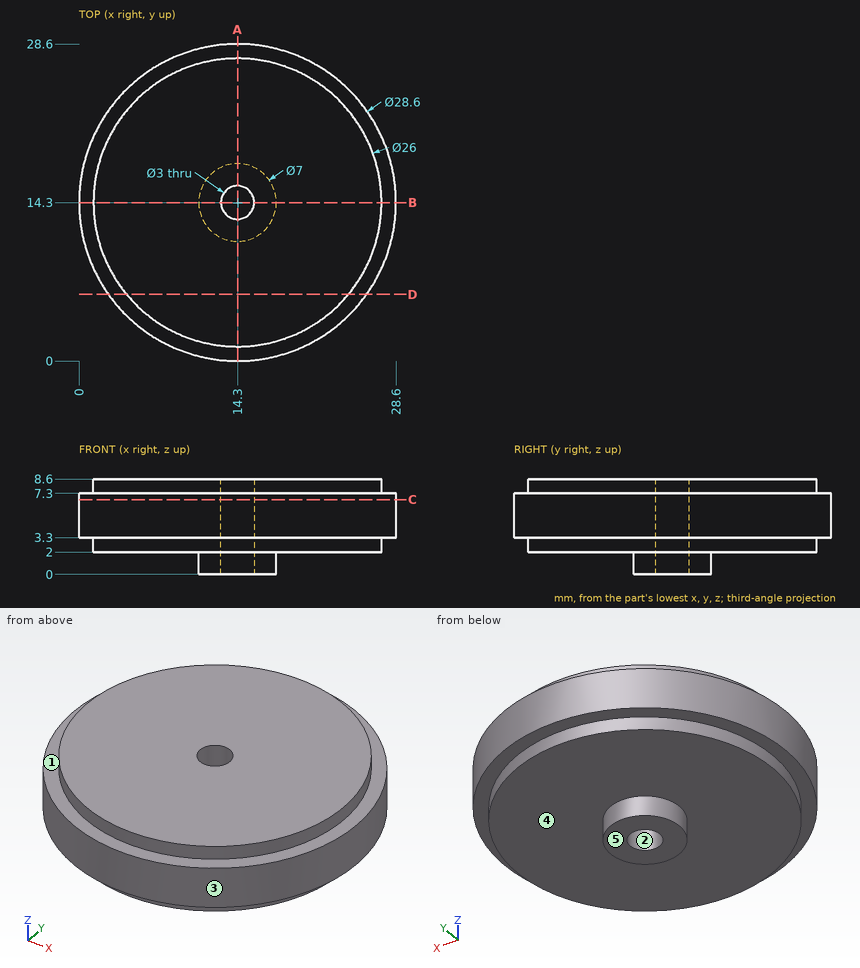
The drawing under review shows one solid part. Ordinate dimensions are in mm from its lowest x, y, z. A direction names the side the tool comes from. Give positions to 0.01 mm unless a question says otherwise; leave off trailing zeros. Write each loop counter-clockwise with the first axis right and the second up, starting at its lowest first coordinate (ties: lowest second). Pieces come first, ordered by that corner, then holes. Notation, with made-up numbers: (-11.75, 15.25) -> (31.25, 15.25) arc R9 ccw to (31.25, 23.25) -> close; hole circle Ø7 at (-14, 29). An arc over 180 degrees is marked (long way). Answer in a Markdown table with one row per item.
(1) Consider section D-D (y = 6). State the section outline as (x, z) points.
Results:
| item | result |
|---|---|
| outline | (2.66, 3.3) -> (4.29, 3.3) -> (4.29, 2) -> (24.31, 2) -> (24.31, 3.3) -> (25.94, 3.3) -> (25.94, 7.3) -> (24.31, 7.3) -> (24.31, 8.6) -> (4.29, 8.6) -> (4.29, 7.3) -> (2.66, 7.3) -> close |
(2) For the marked faces 4 and 5, list the 3-axis set-ups (+Z, -Z, +X, -X, +Y, -Y) from which the entire face can be reached by the end or side of a thin tool; tool diameter is ignored.
Results:
| item | result |
|---|---|
| face 4 | -Z |
| face 5 | -Z, +X, -X, +Y, -Y |
(3) Consider section C-C (z = 6.75). State the section outline as (x, y) points.
Results:
| item | result |
|---|---|
| outline | circle Ø28.6 at (14.3, 14.3); hole circle Ø3 at (14.3, 14.3) |
(4) To check wall thickness, follow probe 1 along Y at (x, z) = (14.3, 6.75); probe 2 along Z at (x, y) = (15, 25.5); probe 3 along Z at (x, y) = (23.75, 3.75). State the ranges of each line that lie inside material, in increasing order.
Results:
| item | result |
|---|---|
| probe 1 | 0 to 12.8, 15.8 to 28.6 |
| probe 2 | 2 to 8.6 |
| probe 3 | 3.3 to 7.3 |
(5) Consider section A-A (x = 14.3). State the section outline as (y, z) points.
Results:
| item | result |
|---|---|
| outline | (0, 3.3) -> (1.3, 3.3) -> (1.3, 2) -> (10.8, 2) -> (10.8, 0) -> (12.8, 0) -> (12.8, 8.6) -> (1.3, 8.6) -> (1.3, 7.3) -> (0, 7.3) -> close; (15.8, 0) -> (17.8, 0) -> (17.8, 2) -> (27.3, 2) -> (27.3, 3.3) -> (28.6, 3.3) -> (28.6, 7.3) -> (27.3, 7.3) -> (27.3, 8.6) -> (15.8, 8.6) -> close |
(6) Mouldability with a two-part tool opening along X and no side actions: class the marked faces 1, 2 and 3 as +X half, -X half, draft (parallel to the pull), parting line (faces both ways), or undercut.
Results:
| item | result |
|---|---|
| face 1 | draft |
| face 2 | undercut |
| face 3 | parting line |
(7) Clearance check with flat-ended pins moving along their axes: pin 1 (5 mm diameter, centred on x = 7, y = 25, fed in from -Z); pin 2 (1.5 mm diameter, centred on y = 21, z = 6.5, fed in from -X); pin 3 (1.5 mm diameter, centred on x = 22, z = 6, fed in from -Y). State where each tip first meets the part, or that it passes through.
Results:
| item | result |
|---|---|
| pin 1 | z = 2 |
| pin 2 | x = 1.3 |
| pin 3 | y = 1.8 |
